CAD build for the part. Positions are in the model's coordinates, mm. A direction names the side the tool comes from. Give positions to 0.01 mm unless a question says otherwise; leave off trailing zeros. Order: outer loops, then holes, each group sorted by start corner. A loop starts at its lowest first (then second) coordinate and runs counter-clockwise, first axis right, second up. Notation, with made-up numbers: (32, -10.5) -> (48, -10.5) arc R35 ccw to (48, 27.5) -> close; hole circle Ø6 at (78, 47.25). An arc over 180 degrees is marked (long way). Answer as CSV lines item,"result".
```python
from build123d import *

# Parameters (mm, degrees)
SKETCH2_R           = 40
SKETCH2_R_2         = 25
SKETCH2_R_3         = 2.1
BOSS_EXTRUDE1_DEPTH = 10
SKETCH4_R           = 30
SKETCH4_R_2         = 25
BOSS_EXTRUDE2_DEPTH = 30
SKETCH5_R           = 30
SKETCH5_R_2         = 1.5
BOSS_EXTRUDE3_DEPTH = 5


with BuildPart() as part:
    # Sketch2 → Boss-Extrude1 (new body)
    with BuildSketch(Plane(origin=(0, 0, 0), x_dir=(1, 0, 0), z_dir=(0, 1, 0))):
        with Locations(Location((0, 0, 0), (0, 0, 270))):
            Circle(SKETCH2_R)
        with Locations(Location((0, 0, 0), (0, 0, 270))):
            Circle(SKETCH2_R_2, mode=Mode.SUBTRACT)
        with Locations(Location((35, 0, 0), (0, 0, 270))):
            Circle(SKETCH2_R_3, mode=Mode.SUBTRACT)
        with Locations(Location((0, -35, 0), (0, 0, 270))):
            Circle(SKETCH2_R_3, mode=Mode.SUBTRACT)
        with Locations(Location((-35, 0, 0), (0, 0, 270))):
            Circle(SKETCH2_R_3, mode=Mode.SUBTRACT)
        with Locations(Location((0, 35, 0), (0, 0, 270))):
            Circle(SKETCH2_R_3, mode=Mode.SUBTRACT)
    extrude(amount=BOSS_EXTRUDE1_DEPTH)

    # Sketch4 → Boss-Extrude2 (add)
    with BuildSketch(Plane(origin=(0, 10, 0), x_dir=(1, 0, 0), z_dir=(0, 1, 0))):
        with Locations(Location((0, 0, 0), (0, 0, 270))):
            Circle(SKETCH4_R)
        with Locations(Location((0, 0, 0), (0, 0, 270))):
            Circle(SKETCH4_R_2, mode=Mode.SUBTRACT)
    extrude(amount=BOSS_EXTRUDE2_DEPTH)

    # Sketch5 → Boss-Extrude3 (add)
    with BuildSketch(Plane(origin=(0, 40, 0), x_dir=(1, 0, 0), z_dir=(0, 1, 0))):
        with Locations(Location((0, 0, 0), (0, 0, 270))):
            Circle(SKETCH5_R)
        with Locations(Location((0, 5, 0), (0, 0, 270))):
            Circle(SKETCH5_R_2, mode=Mode.SUBTRACT)
        with Locations(Location((0, 10, 0), (0, 0, 270))):
            Circle(SKETCH5_R_2, mode=Mode.SUBTRACT)
        with Locations(Location((0, 15, 0), (0, 0, 270))):
            Circle(SKETCH5_R_2, mode=Mode.SUBTRACT)
        with Locations(Location((0, 20, 0), (0, 0, 270))):
            Circle(SKETCH5_R_2, mode=Mode.SUBTRACT)
        with Locations(Location((4.330127019, 2.5, 0), (0, 0, 270))):
            Circle(SKETCH5_R_2, mode=Mode.SUBTRACT)
        with Locations(Location((4.330127019, -2.5, 0), (0, 0, 270))):
            Circle(SKETCH5_R_2, mode=Mode.SUBTRACT)
        with Locations(Location((0, -5, 0), (0, 0, 270))):
            Circle(SKETCH5_R_2, mode=Mode.SUBTRACT)
        with Locations(Location((-4.330127019, -2.5, 0), (0, 0, 270))):
            Circle(SKETCH5_R_2, mode=Mode.SUBTRACT)
        with Locations(Location((-4.330127019, 2.5, 0), (0, 0, 270))):
            Circle(SKETCH5_R_2, mode=Mode.SUBTRACT)
        with Locations(Location((5, 8.660254038, 0), (0, 0, 270))):
            Circle(SKETCH5_R_2, mode=Mode.SUBTRACT)
        with Locations(Location((8.660254038, 5, 0), (0, 0, 270))):
            Circle(SKETCH5_R_2, mode=Mode.SUBTRACT)
        with Locations(Location((10, 0, 0), (0, 0, 270))):
            Circle(SKETCH5_R_2, mode=Mode.SUBTRACT)
        with Locations(Location((8.660254038, -5, 0), (0, 0, 270))):
            Circle(SKETCH5_R_2, mode=Mode.SUBTRACT)
        with Locations(Location((5, -8.660254038, 0), (0, 0, 270))):
            Circle(SKETCH5_R_2, mode=Mode.SUBTRACT)
        with Locations(Location((0, -10, 0), (0, 0, 270))):
            Circle(SKETCH5_R_2, mode=Mode.SUBTRACT)
        with Locations(Location((-5, -8.660254038, 0), (0, 0, 270))):
            Circle(SKETCH5_R_2, mode=Mode.SUBTRACT)
        with Locations(Location((-8.660254038, -5, 0), (0, 0, 270))):
            Circle(SKETCH5_R_2, mode=Mode.SUBTRACT)
        with Locations(Location((-10, 0, 0), (0, 0, 270))):
            Circle(SKETCH5_R_2, mode=Mode.SUBTRACT)
        with Locations(Location((-8.660254038, 5, 0), (0, 0, 270))):
            Circle(SKETCH5_R_2, mode=Mode.SUBTRACT)
        with Locations(Location((-5, 8.660254038, 0), (0, 0, 270))):
            Circle(SKETCH5_R_2, mode=Mode.SUBTRACT)
        with Locations(Location((4.635254916, 14.265847744, 0), (0, 0, 270))):
            Circle(SKETCH5_R_2, mode=Mode.SUBTRACT)
        with Locations(Location((8.816778784, 12.135254916, 0), (0, 0, 270))):
            Circle(SKETCH5_R_2, mode=Mode.SUBTRACT)
        with Locations(Location((12.135254916, 8.816778784, 0), (0, 0, 270))):
            Circle(SKETCH5_R_2, mode=Mode.SUBTRACT)
        with Locations(Location((14.265847744, 4.635254916, 0), (0, 0, 270))):
            Circle(SKETCH5_R_2, mode=Mode.SUBTRACT)
        with Locations(Location((15, 0, 0), (0, 0, 270))):
            Circle(SKETCH5_R_2, mode=Mode.SUBTRACT)
        with Locations(Location((14.265847744, -4.635254916, 0), (0, 0, 270))):
            Circle(SKETCH5_R_2, mode=Mode.SUBTRACT)
        with Locations(Location((12.135254916, -8.816778784, 0), (0, 0, 270))):
            Circle(SKETCH5_R_2, mode=Mode.SUBTRACT)
        with Locations(Location((8.816778784, -12.135254916, 0), (0, 0, 270))):
            Circle(SKETCH5_R_2, mode=Mode.SUBTRACT)
        with Locations(Location((4.635254916, -14.265847744, 0), (0, 0, 270))):
            Circle(SKETCH5_R_2, mode=Mode.SUBTRACT)
        with Locations(Location((0, -15, 0), (0, 0, 270))):
            Circle(SKETCH5_R_2, mode=Mode.SUBTRACT)
        with Locations(Location((-4.635254916, -14.265847744, 0), (0, 0, 270))):
            Circle(SKETCH5_R_2, mode=Mode.SUBTRACT)
        with Locations(Location((-8.816778784, -12.135254916, 0), (0, 0, 270))):
            Circle(SKETCH5_R_2, mode=Mode.SUBTRACT)
        with Locations(Location((-12.135254916, -8.816778784, 0), (0, 0, 270))):
            Circle(SKETCH5_R_2, mode=Mode.SUBTRACT)
        with Locations(Location((-14.265847744, -4.635254916, 0), (0, 0, 270))):
            Circle(SKETCH5_R_2, mode=Mode.SUBTRACT)
        with Locations(Location((-15, 0, 0), (0, 0, 270))):
            Circle(SKETCH5_R_2, mode=Mode.SUBTRACT)
        with Locations(Location((-14.265847744, 4.635254916, 0), (0, 0, 270))):
            Circle(SKETCH5_R_2, mode=Mode.SUBTRACT)
        with Locations(Location((-12.135254916, 8.816778784, 0), (0, 0, 270))):
            Circle(SKETCH5_R_2, mode=Mode.SUBTRACT)
        with Locations(Location((-8.816778784, 12.135254916, 0), (0, 0, 270))):
            Circle(SKETCH5_R_2, mode=Mode.SUBTRACT)
        with Locations(Location((-4.635254916, 14.265847744, 0), (0, 0, 270))):
            Circle(SKETCH5_R_2, mode=Mode.SUBTRACT)
        with Locations(Location((5.176380902, 19.318516526, 0), (0, 0, 270))):
            Circle(SKETCH5_R_2, mode=Mode.SUBTRACT)
        with Locations(Location((10, 17.320508076, 0), (0, 0, 270))):
            Circle(SKETCH5_R_2, mode=Mode.SUBTRACT)
        with Locations(Location((14.142135624, 14.142135624, 0), (0, 0, 270))):
            Circle(SKETCH5_R_2, mode=Mode.SUBTRACT)
        with Locations(Location((17.320508076, 10, 0), (0, 0, 270))):
            Circle(SKETCH5_R_2, mode=Mode.SUBTRACT)
        with Locations(Location((19.318516526, 5.176380902, 0), (0, 0, 270))):
            Circle(SKETCH5_R_2, mode=Mode.SUBTRACT)
        with Locations(Location((20, 0, 0), (0, 0, 270))):
            Circle(SKETCH5_R_2, mode=Mode.SUBTRACT)
        with Locations(Location((19.318516526, -5.176380902, 0), (0, 0, 270))):
            Circle(SKETCH5_R_2, mode=Mode.SUBTRACT)
        with Locations(Location((17.320508076, -10, 0), (0, 0, 270))):
            Circle(SKETCH5_R_2, mode=Mode.SUBTRACT)
        with Locations(Location((14.142135624, -14.142135624, 0), (0, 0, 270))):
            Circle(SKETCH5_R_2, mode=Mode.SUBTRACT)
        with Locations(Location((10, -17.320508076, 0), (0, 0, 270))):
            Circle(SKETCH5_R_2, mode=Mode.SUBTRACT)
        with Locations(Location((5.176380902, -19.318516526, 0), (0, 0, 270))):
            Circle(SKETCH5_R_2, mode=Mode.SUBTRACT)
        with Locations(Location((0, -20, 0), (0, 0, 270))):
            Circle(SKETCH5_R_2, mode=Mode.SUBTRACT)
        with Locations(Location((-5.176380902, -19.318516526, 0), (0, 0, 270))):
            Circle(SKETCH5_R_2, mode=Mode.SUBTRACT)
        with Locations(Location((-10, -17.320508076, 0), (0, 0, 270))):
            Circle(SKETCH5_R_2, mode=Mode.SUBTRACT)
        with Locations(Location((-14.142135624, -14.142135624, 0), (0, 0, 270))):
            Circle(SKETCH5_R_2, mode=Mode.SUBTRACT)
        with Locations(Location((-17.320508076, -10, 0), (0, 0, 270))):
            Circle(SKETCH5_R_2, mode=Mode.SUBTRACT)
        with Locations(Location((-19.318516526, -5.176380902, 0), (0, 0, 270))):
            Circle(SKETCH5_R_2, mode=Mode.SUBTRACT)
        with Locations(Location((-20, 0, 0), (0, 0, 270))):
            Circle(SKETCH5_R_2, mode=Mode.SUBTRACT)
        with Locations(Location((-19.318516526, 5.176380902, 0), (0, 0, 270))):
            Circle(SKETCH5_R_2, mode=Mode.SUBTRACT)
        with Locations(Location((-17.320508076, 10, 0), (0, 0, 270))):
            Circle(SKETCH5_R_2, mode=Mode.SUBTRACT)
        with Locations(Location((-14.142135624, 14.142135624, 0), (0, 0, 270))):
            Circle(SKETCH5_R_2, mode=Mode.SUBTRACT)
        with Locations(Location((-10, 17.320508076, 0), (0, 0, 270))):
            Circle(SKETCH5_R_2, mode=Mode.SUBTRACT)
        with Locations(Location((-5.176380902, 19.318516526, 0), (0, 0, 270))):
            Circle(SKETCH5_R_2, mode=Mode.SUBTRACT)
    extrude(amount=BOSS_EXTRUDE3_DEPTH)


solid = part.part
```
1) Pull direction Z, two halves, no side cores. Call faces 3 (the flat face through (-29, 10, 9)), 4 (the cylindrical face through (0.09, 4.93, 32.9)): pulls with the +Z half, pulls with the -Z half, needs draft (parallel to the pull), parting line crosses it, or undercut.
Data:
face 3,"needs draft"
face 4,"undercut"
2) Band-saw the part on A-A, the plane y = 3. Write the cut outline in (x, z), then the cut area to 3 significant figures.
Data:
outline,"circle Ø80 at (0, 0); hole circle Ø4.2 at (-35, 0); hole circle Ø50 at (0, 0); hole circle Ø4.2 at (0, -35); hole circle Ø4.2 at (0, 35); hole circle Ø4.2 at (35, 0)"
area,"3,010 mm2"
3) Band-saw the part on B-B, the plane z = 34. Write the cut outline in (x, y).
Data:
outline,"(-21.07, 0) -> (-1.85, 0) -> (-1.85, 10) -> (-21.07, 10) -> close; (1.85, 0) -> (21.07, 0) -> (21.07, 10) -> (1.85, 10) -> close"
4) Band-saw the part on D-D, the plane y = 13. Write the cut outline in (x, z), then the cut area to 3 significant figures.
Data:
outline,"circle Ø60 at (0, 0); hole circle Ø50 at (0, 0)"
area,"864 mm2"
5) Wall check: line 1 along X through (y, z) = (43, -2); line 2 along X through (y, z) = (42, -20); line 3 along Y through (x, z) = (35, -7.5). Give the ranges that are in metal, low to high. Write a range as [from, to].
Data:
line 1,"x = [-29.93, -5.74], [-2.92, 2.92], [5.74, 29.93]"
line 2,"x = [-22.36, -6.51], [-3.84, -1.5], [1.5, 3.84], [6.51, 22.36]"
line 3,"y = [0, 10]"
6) Pin check, flat tips, straight feed: P1, Ø1.5, axis at y = 7.5, z = -16, coming from the +X side; P2, Ø2, axis at x = -20, y = 34, coming from the -Z side; P3, Ø4, axis at x = 5.18, z = 19.32, coming from the -Y side. Stop position of each tip, or through.
Data:
P1,"stops at x = 36.98"
P2,"stops at z = -23.22"
P3,"stops at y = 40"
7) Band-saw the part on C-C, the plane z = -23.5. Write the cut outline in (x, y).
Data:
outline,"(-32.37, 0) -> (-8.53, 0) -> (-8.53, 40) -> (8.53, 40) -> (8.53, 0) -> (32.37, 0) -> (32.37, 10) -> (18.65, 10) -> (18.65, 45) -> (-18.65, 45) -> (-18.65, 10) -> (-32.37, 10) -> close"
8) Which spindle directions (+Z, -Z, +X, -X, +Y, -Y) get a long thin tool onto all of the face, cutting with end or side? Do faces 1 (the cylindrical face through (7.509, 19.72, 23.846)), 2 (the cylindrical face through (-12.78, 42.46, 4.44)). Say none if no direction does.
Data:
face 1,"-Y"
face 2,"+Y, -Y"
